For this review, take the finished solid that the model builds, in its own axes (mm). A direction names the side the tool comes from. Give positions to 0.01 mm unless a question says otherwise; leave off trailing zeros. Write each loop counter-clockwise with the first axis right and the second up, starting at its lowest first coordinate (ties: lowest second). Pieces come first, ordered by that corner, then holes. Notation, with made-up numbers: M -17.5,-33 L 32.5,-33 A21 cw 32.5,-24 Z; hole C 40.25,20 d4. An arc over 180 degrees is marked long. Write item = value, one per line.
```python
from build123d import *

# Parameters (mm, degrees)
SKETCH1_W                = 15
SKETCH1_H                = 15.5
BOSS_EXTRUDE1_DEPTH      = 118
BOSS_EXTRUDE2_DEPTH      = 16.2
BOSS_EXTRUDE2_DEPTH_BACK = 134.2


with BuildPart() as part:
    # Sketch1 → Boss-Extrude1 (new body)
    with BuildSketch(Plane.XY):
        Rectangle(SKETCH1_W, SKETCH1_H)
    extrude(amount=BOSS_EXTRUDE1_DEPTH)

    # Sketch2 → Boss-Extrude2 (add, two sides)
    with BuildSketch(Plane.XY.offset(118)) as boss_extrude2_sk:
        with BuildLine():
            Line((-7.5, 7.75), (-7.5, 10.75))
            ThreePointArc((-7.5, 10.75), (0, 18.25), (7.5, 10.75))
            Line((7.5, 10.75), (7.5, 7.75))
            Line((7.5, 7.75), (-7.5, 7.75))
        make_face()
    extrude(amount=BOSS_EXTRUDE2_DEPTH)
    extrude(boss_extrude2_sk.sketch, amount=-BOSS_EXTRUDE2_DEPTH_BACK)


solid = part.part
```
1. We need section A-A, the plane x = 0. Write out the cut boundary in (y, z).
Responses:
outline = M -7.75,0 L 7.75,0 L 7.75,-16.2 L 18.25,-16.2 L 18.25,134.2 L 7.75,134.2 L 7.75,118 L -7.75,118 Z
2. For line 1 along Z through (x, y) = (2.5, 6.75); line 2 along Y through (x, z) = (-5.75, 112.5); line 3 along Y through (x, z) = (-3.5, 82), list the stretches that pass through material, from the lowest coordinate up. Write a range as from..to.
Responses:
line_1 = 0..118
line_2 = -7.75..15.57
line_3 = -7.75..17.38
3. We need section D-D, the plane x = -5.75. Write out the cut boundary in (y, z).
Responses:
outline = M -7.75,0 L 7.75,0 L 7.75,-16.2 L 15.57,-16.2 L 15.57,134.2 L 7.75,134.2 L 7.75,118 L -7.75,118 Z
4. We need section C-C, the plane z = -5.5. Write out the cut boundary in (x, y), then the cut area to 3 significant figures.
Responses:
outline = M -7.5,7.75 L 7.5,7.75 L 7.5,10.75 A7.5 ccw -7.5,10.75 Z
area = 133 mm2
5. Insertion check: P1, Ø5, axis at x = -2, y = 5.5, coming from the +Z side; P2, Ø3, axis at x = -2, z = 69, coming from the +Y side; P3, Ø4.5, axis at x = 3, z = 129, coming from the -Y side; P4, Ø4.5, axis at x = 3, y = 0.5, coming from the -Z side. Each pin has a flat end and moves straight along its axis. Give the tip position at first contact, or say it passes through.
Responses:
P1 = 134.2
P2 = 18.23
P3 = 7.75
P4 = 0
6. Machinability: for faces 1 (the face through (0, 0, 118)), 2 (the face through (0, 7.75, -8)), 3 (the face through (7.5, 2, 60)), which of the approach directions +Z, -Z, +X, -X, +Y, -Y give a long, thin tool a straight path to every point of the face, cutting with its end or side? Answer none if there is none.
Responses:
face_1 = +Z, +X, -X, -Y
face_2 = -Z, +X, -X, -Y
face_3 = +Z, -Z, +X, +Y, -Y
7. We need section B-B, the plane y = -2.25. Write out the cut boundary in (x, z).
Responses:
outline = M -7.5,0 L 7.5,0 L 7.5,118 L -7.5,118 Z
